Verification items for the finished model (mm, model axes). A direction names the side the tool comes from. Coordinates: 2 decimals unless noted, no trailing zeros. Loops run counter-clockwise (first coordinate to the right, second up) from the corner with the lowest first, then second, coordinate; pieces in that order, holes last. Notation, with made-up numbers: (-12.5, -35) - (15.5, -35) arc R22 ccw to (15.5, -10) - close; hole circle Ø6 at (52, 23). An arc over 180 degrees is marked (long way). One line per item, written item: value. Start each with the question number.
(1) Draft check along X on faces 3 (the face through (-19.875, -12.957, 52.675)), 4 (the face through (-13.944, 14.297, 53.986)), 5 (the face through (0, 0, 30)). Enter one of: +X half, -X half, draft (parallel to the pull), parting line (faces both ways), or undercut.
(2) Thickness scan on probe 1 along Z at (x, y) = (15.25, 0); probe 2 along X at (y, z) = (-5.5, 37); probe 3 along Z at (x, y) = (-2, -18). Record the ranges inside material, lowest first. Write a range as [from, to].
(3) Gauge pin test, flat ends, axial feed: P1, Ø7, axis at y = 0, z = 40, coming from the -X side; P2, Ø4, axis at y = -14, z = 54, coming from the +X side; P3, Ø10, axis at x = 0, y = 1, coming from the +Z side; P4, Ø4, axis at x = -10.5, y = 11, coming from the +Z side. Record the tip position at first contact, or that the pin passes through.
(4) Set-up check for faces 1 (the face through (-10, 4, 45)), 2 (the face through (-20, 0, 29)): record each of +Z, -Z, +X, -X, +Y, -Y from which the full face is reachable in a straight line by a thin tool's end or side.
(5) Section check B-B (x = 5.5). Record the boundary of the cut face in (y, z), plus the area to 3 significant figures.
(6) Section check C-C (y = 1.5). Count the separate pieces of the cut face and the enclosed holes in it, plus the area to 3 significant figures.
```python
from build123d import *

# Parameters (mm, degrees)
F0_W          = 40
F0_H          = 40
F1_DEPTH      = 60
F2_W          = 20
F2_H          = 40
F3_DEPTH      = 30
F4_R          = 19.99999
F5_SIZE       = 2
F6_R          = 6
F7_DEPTH      = 56.6
F7_DEPTH_BACK = 25


# Not quite as in the source:
# - a fillet or chamfer is up to 0.001 mm smaller than in the source, because OpenCascade refuses the exact size


with BuildPart() as f1:
    # F0 (on Top) → F1 (new body)
    with BuildSketch(Plane.XY):
        Rectangle(F0_W, F0_H)
    extrude(amount=F1_DEPTH)

    # F2 (on face) → F3 (cut)
    with BuildSketch(Plane.XY.offset(60)):
        Rectangle(F2_W, F2_H)
    extrude(amount=-F3_DEPTH, mode=Mode.SUBTRACT)

    # F4 (radius 20 in the source; OpenCascade refuses exactly that, so slightly less here)
    f4_edges = [f1.edges().sort_by_distance(p)[0] for p in [
        (15, -20, 60),
        (-15, -20, 60),
        (15, 20, 60),
        (-15, 20, 60),
    ]]
    fillet(f4_edges, radius=F4_R)

    # F5
    f5_edges = [f1.edges().sort_by_distance(p)[0] for p in [
        (-20, -20, 20.000005),
        (-20, -14.142139, 54.142139),
        (20, -14.142139, 54.142139),
    ]]
    chamfer(f5_edges, length=F5_SIZE)

    # F6 (on face) → F7 (cut, two sides)
    with BuildSketch(Plane.YZ.offset(20)) as f7_sk:
        with Locations((0, 40)):
            Circle(F6_R)
    extrude(amount=-F7_DEPTH, mode=Mode.SUBTRACT)
    extrude(f7_sk.sketch, amount=F7_DEPTH_BACK, mode=Mode.SUBTRACT)


solid = f1.part
```
Responses:
1. face 3: -X half
1. face 4: draft
1. face 5: undercut
2. probe 1: z = [0, 34], [46, 60]
2. probe 2: x = [-20, -10], [10, 20]
2. probe 3: z = [0, 30]
3. P1: passes through
3. P2: stops at x = 20
3. P3: stops at z = 30
3. P4: stops at z = 57.86
4. face 1: +Z, +Y, -Y
4. face 2: +Z, -Z, -X, +Y, -Y
5. outline: (-20, 0) - (20, 0) - (20, 30) - (-20, 30) - close
5. area: 1,200 mm²
6. separate pieces: 3
6. enclosed holes: 0
6. area: 1,560 mm²
